```python
from build123d import *

# Parameters (mm, degrees)
SKETCH1_R                = 40
SKETCH1_R_2              = 10
BOSS_EXTRUDE1_DEPTH      = 12.5
SKETCH2_R                = 22.5
CUT_EXTRUDE1_DEPTH       = 10
SKETCH3_R                = 3
CUT_EXTRUDE2_DEPTH       = 16
CIRPATTERN1_COUNT        = 5
SKETCH4_R                = 11
SKETCH4_R_2              = 10
BOSS_EXTRUDE2_DEPTH      = 2
BOSS_EXTRUDE2_DEPTH_BACK = 7


with BuildPart() as part:
    # Sketch1 → Boss-Extrude1 (new body, symmetric)
    with BuildSketch(Plane.XY):
        Circle(SKETCH1_R)
        Circle(SKETCH1_R_2, mode=Mode.SUBTRACT)
    extrude(amount=BOSS_EXTRUDE1_DEPTH, both=True)

    # Sketch2 → Cut-Extrude1 (cut)
    with BuildSketch(Plane.XY.offset(12.5)):
        Circle(SKETCH2_R)
    cut_extrude1 = extrude(amount=-CUT_EXTRUDE1_DEPTH, mode=Mode.SUBTRACT)

    # Mirror1: Cut-Extrude1 across plane
    add(cut_extrude1.mirror(Plane.XY), mode=Mode.SUBTRACT)

    # Sketch3 → Cut-Extrude2 (cut, through all)
    with BuildSketch(Plane.XY.offset(2.5)):
        with Locations((0, 17)):
            Circle(SKETCH3_R)
    cut_extrude2 = extrude(amount=-CUT_EXTRUDE2_DEPTH, mode=Mode.SUBTRACT)

    # CirPattern1: Cut-Extrude2 ×5 about axis
    cirpattern1_axis = Axis((0, 0, 0), (0, 0, 1))
    for i in range(1, CIRPATTERN1_COUNT):
        add(cut_extrude2.rotate(cirpattern1_axis, i * 360 / CIRPATTERN1_COUNT), mode=Mode.SUBTRACT)

    # Sketch4 → Boss-Extrude2 (add, two sides)
    with BuildSketch(Plane.XY.offset(2.5)) as boss_extrude2_sk:
        Circle(SKETCH4_R)
        Circle(SKETCH4_R_2, mode=Mode.SUBTRACT)
    extrude(amount=BOSS_EXTRUDE2_DEPTH)
    extrude(boss_extrude2_sk.sketch, amount=-BOSS_EXTRUDE2_DEPTH_BACK)

    # Sketch5 → Cut-Revolve1 (revolve, cut)
    with BuildSketch(Plane(origin=(0, 0, 0), x_dir=(1, 0, 0), z_dir=(0, 1, 0))):
        Polygon((-40, 9.5), (-34, 6.035898385), (-34, -6.035898385), (-40, -9.5), align=None)
    revolve(axis=Axis((0, 0, 0), (0, 0, -1)), mode=Mode.SUBTRACT)


solid = part.part
```
CAD build for the part. Positions are in the model's coordinates, mm. A direction names the side the tool comes from. Give positions to 0.01 mm unless a question says otherwise; leave off trailing zeros. Write each loop counter-clockwise with the first axis right and the second up, starting at its lowest first coordinate (ties: lowest second). Pieces come first, ordered by that corner, then holes. Notation, with made-up numbers: M 87.25,-32 L 119.25,-32 A7 ccw 119.25,-19 Z; hole C 54.25,-1 d8. An arc over 180 degrees is marked long. Return JSON: item names as keys, results as strings. Group by question number.
(1) Flat gauge pins, fed straight in: pin 1 Ø5 at (x, z) = (-9, -7) entering from -Y; pin 2 Ø3 at (x, z) = (11, 3) entering from -Y; pin 3 Ø2 at (x, y) = (11.5, 7) entering from -Z; pin 4 Ø3.5 at (x, y) = (-16.17, 5.25) entering from +Z. Where does each tip first touch, or does it go through?
(2) Mould opens along Z. For faces 6 (the face through (-18.28, 28.67, 0.08)), 7 (the face through (17.413, 7.983, 0.035)), 8 (the face through (10, 5, 2.5)) say: pulls with the +Z half, pulls with the -Z half, needs draft (parallel to the pull), parting line crosses it, or undercut.
(3) Band-saw the part on C-C (z = -8). Give the cut face in (x, y), and give its area (3 significant figures).
(4) Band-saw the part on B-B (x = 0). State how many separate pieces and enclosed holes the cut face has, and give its area (3 significant figures).
(5) Drill centre lines: L1, parallel to Y at x = 0, z = -0.45; L2, parallel to Y at x = 0, z = -3.65; L3, parallel to Z at x = 10.5, y = -2. Where is each one in solid material? Low to high. Write a range as [from, to].
(6) 3-axis set-ups, long thin cutter, end or side, ignore diameter. For faces 1 (the face through (17, -17, -12.5)), 2 (the face through (-32.7, 10.3, -6.2)), 3 (the face through (10, 5, -2.5)), 4 (the face through (-0.65, 14.07, 0.04)), 5 (the face through (10.382, -19.961, 7.57)): which of +Z, -Z, +X, -X, +Y, -Y reach the whole face in a straight line?
Entries:
{
 "1": {"pin 1": "stops at y = -39.01", "pin 2": "stops at y = -32.65", "pin 3": "stops at z = -2.5", "pin 4": "passes through"},
 "2": {"face 6": "undercut", "face 7": "needs draft", "face 8": "pulls with the +Z half"},
 "3": {"outline": "C 0,0 d74.8; hole C 0,0 d45", "area": "2,800 mm^2"},
 "4": {"separate pieces": "3", "enclosed holes": "0", "area": "792 mm^2"},
 "5": {"L1": "y = [-34, -10], [10, 14], [20, 34]", "L2": "y = [-34, -22.5], [-11, -10], [10, 11], [22.5, 34]", "L3": "z = [-4.5, 4.5]"},
 "6": {"face 1": "-Z, +X, -X, +Y, -Y", "face 2": "none", "face 3": "-Z", "face 4": "+Z, -Z", "face 5": "+Z"}
}
